Input: dimensioned drawing with shaded views. Units: mm. Origin: part minimum x, y, z. Round coordinates to 2 decimals unless told otherwise and drop trailing zeros. Loops run counter-clockwise (first coordinate to the right, second up) from the corner with the lowest first, then second, coordinate; pieces in that order, holes last. Notation, with made-up numbers: (28, 38.25) - (53, 38.25) arc R27 cw to (53, 56.25) - close; hole circle Ø7 at (-9.75, 5). An arc over 180 degrees is marked (long way). One line per question, with ' | ' between items.
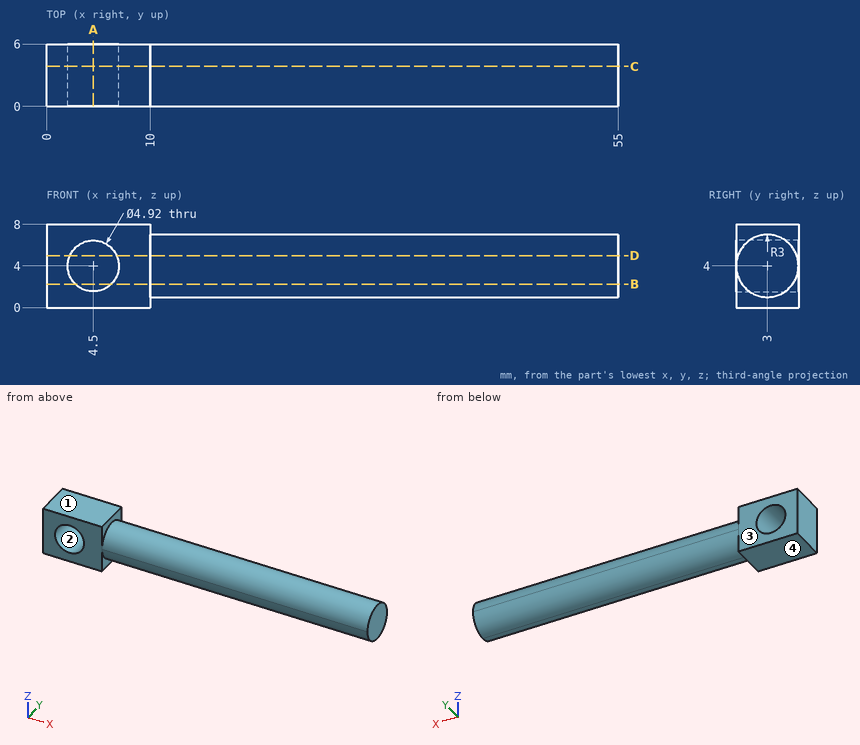
1. Section query D-D, the plane z = 5. Return loops of the section in (x, y).
Worked out:
outline: (0, 0) - (2.25, 0) - (2.25, 6) - (0, 6) - close; (6.75, 0) - (10, 0) - (10, 0.17) - (55, 0.17) - (55, 5.83) - (10, 5.83) - (10, 6) - (6.75, 6) - close
2. Section query A-A, the plane x = 4.5. Return loops of the section in (y, z).
Worked out:
outline: (0, 0) - (6, 0) - (6, 1.54) - (0, 1.54) - close; (0, 6.46) - (6, 6.46) - (6, 8) - (0, 8) - close
3. Section query C-C, the plane y = 3.85. Return loops of the section in (x, z), plus the area to 3 significant figures.
Worked out:
outline: (0, 0) - (10, 0) - (10, 1.12) - (55, 1.12) - (55, 6.88) - (10, 6.88) - (10, 8) - (0, 8) - close; hole circle Ø4.92 at (4.5, 4) | area: 320 mm2
4. Material intervals for probe 1 along X at (y, z) = (4, 4); probe 2 along X at (y, z) = (3.15, 3.5); probe 3 along Z at (x, y) = (6, 4.1), sorted ascending.
Worked out:
probe 1: x = 0 to 2.04, 6.96 to 55 | probe 2: x = 0 to 2.09, 6.91 to 55 | probe 3: z = 0 to 2.05, 5.95 to 8
5. Contact query for flat-ended pins moving along their axis: P1, Ø1, axis at x = 49.5, y = 3, coming from the +Z side; P2, Ø1.5, axis at x = 38.5, z = 1, coming from the -Y side; P3, Ø1, axis at x = 23.5, y = 4.5, coming from the -Z side. Output: stop coordinate, or through.
Worked out:
P1: stops at z = 7 | P2: stops at y = 1.02 | P3: stops at z = 1.17
6. Section query B-B, the plane z = 2.25. Return loops of the section in (x, y).
Worked out:
outline: (0, 0) - (2.77, 0) - (2.77, 6) - (0, 6) - close; (6.23, 0) - (10, 0) - (10, 0.56) - (55, 0.56) - (55, 5.44) - (10, 5.44) - (10, 6) - (6.23, 6) - close
7. Mould query, pull axis Z, two halves, no side actions, for the marked faces 1, 2, 3 and 4. Classes: released by +Z, released by -Z, zero draft, split by the parting line, or undercut.
Worked out:
face 1: released by +Z | face 2: undercut | face 3: zero draft | face 4: released by -Z
